Geometry check sheet. Reference: the model listing, model coordinates, mm. Face numbers are marked on the shaded views. A direction names the side the tool comes from. Round coordinates to 2 decimals unless told otherwise and drop trailing zeros. Write each loop counter-clockwise with the first axis right and the second up, starting at its lowest first coordinate (ties: lowest second). Pieces come first, ordered by that corner, then holes. Notation, with made-up numbers: M 38,1 L 76,1 A21 cw 76,15 Z; hole C -3,-17.75 d1. An arc over 180 degrees is marked long. Use a Markdown table: item, result.
```python
from build123d import *
from build123d.topology import SkipClean

# Parameters (mm, degrees)
SKETCH_1_R      = 35
SKETCH_1_R_2    = 21.25
EXTRUDE_1_DEPTH = 2
SKETCH_1_3_R    = 21.25
EXTRUDE_2_DEPTH = 24


with BuildPart() as part:
    # Sketch 1 → Extrude 1 (new body)
    # profile 1 of 2: a face of its own
    with BuildSketch(Plane(origin=(0, 0, 0), x_dir=(1, 0, 0), z_dir=(0, 1, 0))):
        with Locations(Location((0, 0, 0), (0, 0, 270))):
            Circle(SKETCH_1_R)
        Circle(SKETCH_1_R_2, mode=Mode.SUBTRACT)
    # profile 2 of 2: a face of its own
    with BuildSketch(Plane(origin=(0, 0, 0), x_dir=(1, 0, 0), z_dir=(0, 1, 0))):
        Circle(SKETCH_1_R_2)
    extrude(amount=EXTRUDE_1_DEPTH)

    # Sketch 1_3 → Extrude 2 (add)
    with BuildSketch(Plane(origin=(0, 0, 0), x_dir=(1, 0, 0), z_dir=(0, 1, 0))):
        with Locations(Location((0, 0, 0), (0, 0, 270))):
            Circle(SKETCH_1_3_R)
    extrude(amount=EXTRUDE_2_DEPTH)

    # Sketch 2 → Revolve 1 (revolve)
    with SkipClean():  # the faces are left unmerged after this step: merging them gives an invalid solid
        with BuildSketch(Plane.XY):
            with BuildLine():
                ThreePointArc((12.7, 18.3), (0, 31), (-12.7, 18.3))
                Line((-12.7, 18.3), (12.7, 18.3))
            make_face()
            with BuildLine():
                Line((12.7, 18.3), (-12.7, 18.3))
                ThreePointArc((-12.7, 18.3), (0, 5.6), (12.7, 18.3))
            make_face()
        revolve(axis=Axis((-1000, 18.3, 0), (1, 0, 0)))


solid = part.part
```
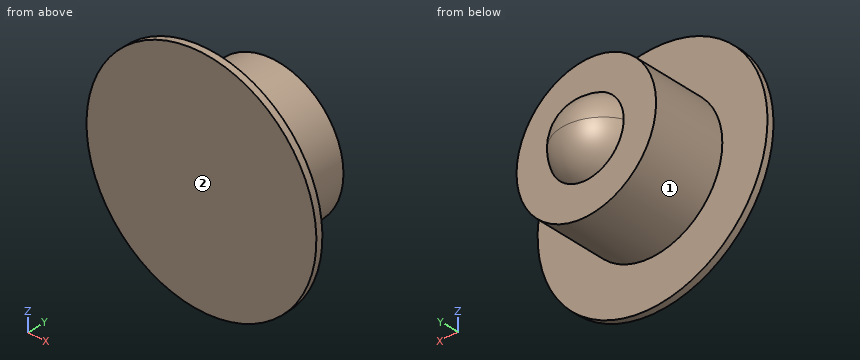
Item 1: Cross-section at A-A, the plane x = -9.5. Record the cut outline in (y, z), and give its area (3 significant figures).
Outcome:
| item | result |
|---|---|
| outline | M 0,-33.69 L 2,-33.69 L 2,-19.01 L 24,-19.01 L 24,-6.21 A8.43 ccw 24,6.21 L 24,19.01 L 2,19.01 L 2,33.69 L 0,33.69 Z |
| area | 995 mm2 |
Item 2: Cross-section at D-D, the plane x = -17. Record the cut outline in (y, z).
Outcome:
| item | result |
|---|---|
| outline | M 0,-30.59 L 2,-30.59 L 2,-12.75 L 24,-12.75 L 24,12.75 L 2,12.75 L 2,30.59 L 0,30.59 Z |
Item 3: Cross-section at C-C, the plane z = -15. Record the cut outline in (x, y).
Outcome:
| item | result |
|---|---|
| outline | M -31.62,0 L 31.62,0 L 31.62,2 L 15.05,2 L 15.05,24 L -15.05,24 L -15.05,2 L -31.62,2 Z |
Item 4: Go/stop test with flat-tipped pins: pin 1 (12 mm diameter, centred on x = -11.5, z = 26.5, fed in from +Y); pin 2 (3 mm diameter, centred on x = -4.5, z = -9.5, fed in from -Y); pin 3 (1 mm diameter, centred on x = 26.5, z = 25.5, fed in from -Y); pin 4 (10 mm diameter, centred on y = 9, z = 14.5, fed in from +X). Record where each tip stops, or that it passes through.
Outcome:
| item | result |
|---|---|
| pin 1 | stops at y = 2 |
| pin 2 | stops at y = 0 |
| pin 3 | passes through |
| pin 4 | stops at x = 19.01 |
Item 5: Material ranges on line 1 along Y through (x, z) = (-19, -19); line 2 along Z through (x, y) = (0.5, 12); line 3 along Y through (x, z) = (-9.5, -12.5), recorded low to high. Write a range as from..to.
Outcome:
| item | result |
|---|---|
| line 1 | y = 0..2 |
| line 2 | z = -21.24..21.24 |
| line 3 | y = 0..24 |
Item 6: Access from +Z, -Z, +X, -X, +Y, -Y to the whole of each face (thin tool, end or side, straight path). Record for the marked faces 1 and 2.
Outcome:
| item | result |
|---|---|
| face 1 | +Y |
| face 2 | +Z, -Z, +X, -X, -Y |
Item 7: Cross-section at B-B, the plane y = 22.5. Record the cut outline in (x, z), and give its area (3 significant figures).
Outcome:
| item | result |
|---|---|
| outline | C 0,0 d42.5 |
| area | 1,420 mm2 |
